```python
from build123d import *

# Parameters (mm, degrees)
F0_R          = 28
F0_R_2        = 26.05
F1_DEPTH      = 30
F2_START      = -10
F2_DEPTH      = 30
F3_START      = -20
F3_DEPTH      = 30
F5_DEPTH      = 1
F5_DEPTH_BACK = 1
F6_DEPTH      = 50
F7_DEPTH      = 150.7
F8_DEPTH      = 50


with BuildPart() as f1:
    # F0 (on Top) → F1 (new body)
    with BuildSketch(Plane.XY):
        with Locations((58, 0)):
            Circle(F0_R)
        with Locations((58, 0)):
            Circle(F0_R_2, mode=Mode.SUBTRACT)
        with Locations((58, 0)):
            Circle(F0_R_2)
    extrude(amount=-F1_DEPTH)



with BuildPart() as f2:
    # F0 (on Top) → F2 (new body)
    with BuildSketch(Plane.XY.offset(F2_START)):
        Circle(F0_R)
        Circle(F0_R_2, mode=Mode.SUBTRACT)
        Circle(F0_R_2)
    extrude(amount=-F2_DEPTH)


with BuildPart() as f3:
    # F0 (on Top) → F3 (new body)
    with BuildSketch(Plane.XY.offset(F3_START)):
        with Locations((-58, 0)):
            Circle(F0_R)
        with Locations((-58, 0)):
            Circle(F0_R_2, mode=Mode.SUBTRACT)
        with Locations((-58, 0)):
            Circle(F0_R_2)
    extrude(amount=-F3_DEPTH)


with BuildPart() as f1_1:
    add(f1.part)

    add(f2.part)  # F5 merges F2

    add(f3.part)  # F5 merges F3
    # F4 (on Front) → F5 (join, two sides)
    with BuildSketch(Plane.XZ) as f5_sk:
        Polygon((91.4459181696, -3.3011357271), (-90.1017620827, -34.3922948223), (-90.1017620827, -39.6512281582), (91.4459181696, -8.560069063), align=None)
    extrude(amount=F5_DEPTH)
    extrude(f5_sk.sketch, amount=-F5_DEPTH_BACK)

    # F0 (on Top) → F6 (cut)
    with BuildSketch(Plane.XY):
        with Locations((-58, 0)):
            Circle(F0_R_2)
    extrude(amount=-F6_DEPTH, mode=Mode.SUBTRACT)

    # F0 (on Top) → F7 (cut)
    with BuildSketch(Plane.XY):
        Circle(F0_R_2)
    extrude(amount=-F7_DEPTH, mode=Mode.SUBTRACT)

    # F0 (on Top) → F8 (cut)
    with BuildSketch(Plane.XY):
        with Locations((58, 0)):
            Circle(F0_R_2)
    extrude(amount=-F8_DEPTH, mode=Mode.SUBTRACT)


solid = f1_1.part
```
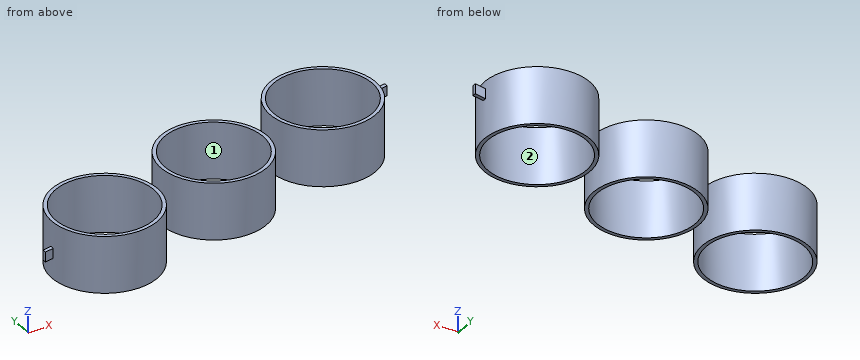
Part model, mm, in its own coordinate system. Face numbers are marked on the shaded views. Round coordinates to 2 decimals unless told otherwise and drop trailing zeros. Loops run counter-clockwise (first coordinate to the right, second up) from the corner with the lowest first, then second, coordinate; pieces in that order, holes last. Notation, with made-up numbers: (47, 73.5) -> (82, 73.5) arc R13 cw to (82, 96.5) -> close; hole circle Ø11 at (66, -32). An arc over 180 degrees is marked (long way). Use a Markdown table: item, result.
1) Cut at D-D, the plane x = 6. List the corners of the cut face in (y, z), and give its area (3 significant figures).
The answers:
| item | result |
|---|---|
| outline | (-27.35, -40) -> (-25.35, -40) -> (-25.35, -10) -> (-27.35, -10) -> close; (25.35, -40) -> (27.35, -40) -> (27.35, -10) -> (25.35, -10) -> close |
| area | 120 mm2 |
2) Probe line 1 (Y direction, x = 0, z = -24.5); line 2 (X direction, y = -14.5, z = -25); line 3 (X direction, y = 20, z = -12). List the from-to ranges inside material, lowest first. Write a range as [from, to].
The answers:
| item | result |
|---|---|
| line 1 | y = [-28, -26.05], [26.05, 28] |
| line 2 | x = [-81.95, -79.64], [-36.36, -34.05], [-23.95, -21.64], [21.64, 23.95], [34.05, 36.36], [79.64, 81.95] |
| line 3 | x = [-19.6, -16.69], [16.69, 19.6], [38.4, 41.31], [74.69, 77.6] |
3) Cut at B-B, the plane x = -58. List the corners of the cut face in (y, z).
The answers:
| item | result |
|---|---|
| outline | (-28, -50) -> (-26.05, -50) -> (-26.05, -20) -> (-28, -20) -> close; (26.05, -50) -> (28, -50) -> (28, -20) -> (26.05, -20) -> close |
4) Drop flat-ended pins along their axis: pin 1 Ø5 at (x, z) = (24, -9) entering from -Y; pin 2 Ø10 at (x, z) = (16.5, -11) entering from +Y; pin 3 Ø4 at (y, z) = (15, -14) entering from +X. Give the stop position or say it passes through.
The answers:
| item | result |
|---|---|
| pin 1 | stops at y = -17.68 |
| pin 2 | stops at y = 25.53 |
| pin 3 | stops at x = 82.8 |
5) Cut at A-A, the plane z = -37. List the corners of the cut face in (x, y).
The answers:
| item | result |
|---|---|
| outline | (-90.1, -1) -> (-85.98, -1) arc R28 ccw (long way) to (-85.98, 1) -> (-90.1, 1) -> close; circle Ø56 at (0, 0); hole circle Ø52.1 at (-58, 0); hole circle Ø52.1 at (0, 0) |
6) Pull direction X, two halves, no side cores. Call the marked faces 1 and 2: pulls with the +X half, pulls with the -X half, needs draft (parallel to the pull), parting line crosses it, or undercut.
The answers:
| item | result |
|---|---|
| face 1 | undercut |
| face 2 | undercut |
7) Cut at C-C, the plane y = -14.5. List the corners of the cut face in (x, z), and give its area (3 significant figures).
The answers:
| item | result |
|---|---|
| outline | (-81.95, -50) -> (-79.64, -50) -> (-79.64, -20) -> (-81.95, -20) -> close; (-36.36, -50) -> (-34.05, -50) -> (-34.05, -20) -> (-36.36, -20) -> close; (-23.95, -40) -> (-21.64, -40) -> (-21.64, -10) -> (-23.95, -10) -> close; (21.64, -40) -> (23.95, -40) -> (23.95, -10) -> (21.64, -10) -> close; (34.05, -30) -> (36.36, -30) -> (36.36, 0) -> (34.05, 0) -> close; (79.64, -30) -> (81.95, -30) -> (81.95, 0) -> (79.64, 0) -> close |
| area | 416 mm2 |
